Input: part model. Units: mm. Frame: model coordinates. A direction names the side the tool comes from. Give positions to 0.01 mm unless a question says otherwise; leave off trailing zeros. Loops run counter-clockwise (first coordinate to the right, second up) from the corner with the lowest first, then second, coordinate; pieces in that order, holes last. Notation, with made-up numbers: (-12, 44.5) - (30, 44.5) arc R7 cw to (30, 52.5) - close; hole circle Ø4 at (86, 59.25). An arc over 180 degrees is marked (long way). One line per item, written item: value.
Autodesk Inventor part; units mm, degrees
ref_plane "YZ Plane" through (0, 0, 0) normal (1, 0, 0) x (0, 1, 0)
ref_plane "XZ Plane" through (0, 0, 0) normal (0, 1, 0) x (-1, 0, 0)
ref_plane "XY Plane" through (0, 0, 0) normal (0, 0, 1) x (1, 0, 0)
sketch "Sketch1" plane through (0, 0, 0) normal (0, 0, 1) x (1, 0, 0)
  arc A0 (-0.7406, 7.8652) -> (0.7406, 7.8652) centre (0, 0) ccw
  line L0 (15, 17.5) -> (15, -17.5)
  line L1 (15, -17.5) -> (-15, -17.5)
  line L2 (-15, -17.5) -> (-15, 17.5)
  line L3 (-15, 17.5) -> (15, -17.5) construction
  line L4 (15, 17.5) -> (-15, -17.5) construction
  line L5 (-0.7406, 7.8652) -> (-0.7406, 17.5)
  line L6 (0.7406, 7.8652) -> (0.7406, 17.5)
  line L7 (-15, 17.5) -> (-0.7406, 17.5)
  line L8 (0.7406, 17.5) -> (15, 17.5)
  dimension "d0" = 15.8
  dimension "d1" = 30
  dimension "d2" = 35
  dimension "d26" = 35
extrude "Extrusion1" add sketch "Sketch1" along normal blind 25
sketch "Sketch2" plane through (-15, -17.5, 0) normal (0, -1, 0) x (1, 0, 0)
  line L0 (15, 0) -> (15, 25)
  line L1 (7.1, 25) -> (22.9, 25)
  line L2 (45, 32.5) -> (-15, 32.5)
  line L3 (-15, 32.5) -> (-15, -7.5)
  line L4 (-15, -7.5) -> (45, -7.5)
  line L5 (45, -7.5) -> (45, 32.5)
  line L6 (45, 32.5) -> (-15, -7.5) construction
  line L7 (-15, 32.5) -> (45, -7.5) construction
  point P0 (15.7406, 25)
  point P1 (14.2594, 25)
  point P2 (15, 12.5)
  dimension "d7" = 60
  dimension "d8" = 40
extrude "Extrusion2" add sketch "Sketch2" along normal blind 6
sketch "Sketch4" plane through (-15, -23.5, 0) normal (0, -1, 0) x (1, 0, 0)
  line L0 (-15, 32.5) -> (-15, -7.5)
  line L1 (45, -7.5) -> (45, 32.5)
  line L2 (-15, -1) -> (45, -1)
  line L3 (-15, 6) -> (45, 6)
  line L4 (-15, 19) -> (45, 19)
  line L5 (-15, 26) -> (45, 26)
  line L6 (-15, -1) -> (-15, 6)
  line L7 (-15, 19) -> (-15, 26)
  line L8 (45, 26) -> (45, 19)
  line L9 (45, 6) -> (45, -1)
  point P0 (15, 0)
extrude "Extrusion3" add sketch "Sketch4" along normal blind 1.5 contours L5 L1 L4 L0 | L3 L1 L2 L0
sketch "Sketch5" plane through (-15, -25, 0) normal (0, -1, 0) x (1, 0, 0)
  line L0 (-14.5701, -1.0846) -> (0, 6)
  line L1 (45, 6) -> (-15, 6)
  line L2 (0, 0) -> (0, 25)
  line L3 (-15, 19) -> (45, 19)
  line L4 (-15, 19) -> (0, 26.2937)
  line L5 (15, 0) -> (15, 25)
  line L6 (7.1, 25) -> (22.9, 25)
  line L7 (44.5701, -1.0846) -> (30, 6)
  line L8 (45, 19) -> (30, 26.2937)
  point P0 (-7.285, 2.4577)
  point P1 (-7.5, 22.6468)
  point P2 (15.7406, 25)
  point P3 (14.2594, 25)
  point P4 (37.285, 2.4577)
  point P5 (37.5, 22.6468)
hole "Hole1" at (-22.285, -25, 2.4577) at (-22.5, -25, 22.6468) at (22.285, -25, 2.4577) at (22.5, -25, 22.6468) direction (0, 1, 0) diameter 5.5 end through all counterbore diameter 10 counterbore depth 1.5
sketch "Sketch6" plane through (-15, 17.5, 0) normal (-1, 0, 0) x (0, 0, 1)
  line L0 (25, 0) -> (25, -35)
  line L1 (0, -9.6348) -> (25, -9.6348)
  line L2 (25, 0) -> (0, -9.6348)
  point P0 (0, -17.5)
  point P1 (12.5, -4.8174)
hole "Hole2" at (-15, 12.6826, 12.5) direction (1, 0, 0) diameter 4.5 end through all
fillet "Fillet1" radius 2 10 edges at (30, -20.5, -7.5) (-30, -20.5, -7.5) (-15, 17.5, 12.5) (-7.8703, 17.5, 0) (7.8703, 17.5, 0) (7.8703, 17.5, 25) (-7.8703, 17.5, 25) (15, 17.5, 12.5) (30, -20.5, 32.5) (-30, -20.5, 32.5)
properties part number "CarroZ - FusoZ"
Item 1: Material intervals for L1, parallel to Z at x = 22.5, y = -20.6; L2, parallel to X at y = 14.5, z = 5; L3, parallel to Y at x = 5.25, z = 12.5, sorted ascending.
Verdict:
L1: z = -7.5 to -0.28, 5.2 to 19.9, 25.4 to 32.5
L2: x = -15 to -0.74, 0.74 to 15
L3: y = -23.5 to -5.9, 5.9 to 10.43, 14.93 to 17.5
Item 2: Section D-D, the plane z = 11.5. Output: boundary loops of the cut face in (x, y).
Verdict:
outline: (-30, -23.5) - (30, -23.5) - (30, -17.5) - (15, -17.5) - (15, 10.67) - (0.74, 10.67) - (0.74, 7.87) arc R7.9 cw (long way) to (-0.74, 7.87) - (-0.74, 10.67) - (-15, 10.67) - (-15, -17.5) - (-30, -17.5) - close; (-15, 14.7) - (-0.74, 14.7) - (-0.74, 17.5) - (-13, 17.5) arc R2 ccw to (-15, 15.5) - close; (0.74, 14.7) - (15, 14.7) - (15, 15.5) arc R2 ccw to (13, 17.5) - (0.74, 17.5) - close
Item 3: Section C-C, the plane x = -5. Output: boundary loops of the cut face in (y, z).
Verdict:
outline: (-25, -1) - (-23.5, -1) - (-23.5, -7.5) - (-17.5, -7.5) - (-17.5, 0) - (-6.12, 0) - (-6.12, 25) - (-17.5, 25) - (-17.5, 32.5) - (-23.5, 32.5) - (-23.5, 26) - (-25, 26) - (-25, 19) - (-23.5, 19) - (-23.5, 6) - (-25, 6) - close; (6.12, 0) - (15.5, 0) arc R2 ccw to (17.5, 2) - (17.5, 23) arc R2 ccw to (15.5, 25) - (6.12, 25) - close; hole circle Ø4.5 at (12.68, 12.5)
Item 4: Section A-A, the plane y = 0. Output: boundary loops of the cut face in (x, z), and give its area (3 significant figures).
Verdict:
outline: (-15, 0) - (-7.9, 0) - (-7.9, 25) - (-15, 25) - close; (7.9, 0) - (15, 0) - (15, 25) - (7.9, 25) - close
area: 355 mm^2
Item 5: Section B-B, the plane z = 17.5. Output: boundary loops of the cut face in (x, y), and give its area (3 significant figures).
Verdict:
outline: (-30, -23.5) - (30, -23.5) - (30, -17.5) - (15, -17.5) - (15, 15.5) arc R2 ccw to (13, 17.5) - (0.74, 17.5) - (0.74, 7.87) arc R7.9 cw (long way) to (-0.74, 7.87) - (-0.74, 17.5) - (-13, 17.5) arc R2 ccw to (-15, 15.5) - (-15, -17.5) - (-30, -17.5) - close
area: 1,200 mm^2
Item 6: Draft query along X for faces 1 (the face through (0, -23.5, 13)), 2 (the face through (-29.4, -20.54, 31.93)), 3 (the face through (7, 17.5, 12)). Return one class per face: pulls with the +X half, pulls with the -X half, needs draft (parallel to the pull), parting line crosses it, or undercut.
Verdict:
face 1: undercut
face 2: pulls with the -X half
face 3: needs draft
Item 7: Access query for faces 4 (the face through (-0.741, 13, 10)), 5 (the face through (-17.502, -24.24, 22.495)), 6 (the face through (15, -1, 12)). Directions: +Z, -Z, +X, -X, +Y, -Y. A direction counts if a zero-diameter tool reaches every point of the face in a straight line with its end or side. Return the directions, or none.
Verdict:
face 4: +Z, -Z, +Y
face 5: -Y
face 6: +Z, -Z, +X, +Y
Item 8: Pin query (flat end, axial travel): P1, Ø24, axis at x = -6, y = -3, coming from the -Z side; P2, Ø5, axis at y = -2.5, z = 27, coming from the -X side; P3, Ø1.6, axis at x = -27.5, y = -24.5, coming from the +Z side; P4, Ø2, axis at y = 1, z = 27, coming from the +X side. Return the tip coordinate at first contact, or that it passes through.
Verdict:
P1: stops at z = 0
P2: stops at x = -15
P3: stops at z = 26
P4: passes through
